Design review of the part shown in the three views and the two pictorial views. Dimensions are in mm from the part's minimum x, y and z. A direction names the side the tool comes from. Give positions to 0.01 mm unless a question says otherwise; leave off trailing zeros. Loops run counter-clockwise (first coordinate to the right, second up) from the corner with the lowest first, then second, coordinate; pieces in that order, holes last. Notation, with made-up numbers: (-26.75, 32) -> (31.25, 32) arc R21 ccw to (31.25, 65) -> close; hole circle Ø6 at (83.5, 1). An arc over 180 degrees is marked (long way). One line per question, with ' | ' between items. Start each with the question number.
(1) Consider section B-B (y = 3). Write out the cut boundary in (x, z).
(2) Insertion check: P1, Ø1.5, axis at x = 10, y = 2, coming from the -Z side; P2, Ø2, axis at x = 3.5, z = 2.5, coming from the -Y side. Each pin has a flat end and moves straight along its axis. Give the tip position at first contact, or say it passes through.
(3) Tool access review of the marked faces 1 and 2: name each direction out of +Z, -Z, +X, -X, +Y, -Y from which nothing blocks a thin tool from reaching the whole face with its end or side.
(4) Consider section C-C (y = 6). Write out the cut boundary in (x, z).
(5) Wall thickness on probe 1 along Y at (x, z) = (7.75, 10.25); probe 2 along Z at (x, y) = (5.5, 4.75); probe 3 along Y at (x, z) = (1.25, 8.75): over which ranges is each line inside the solid? List them lowest first.
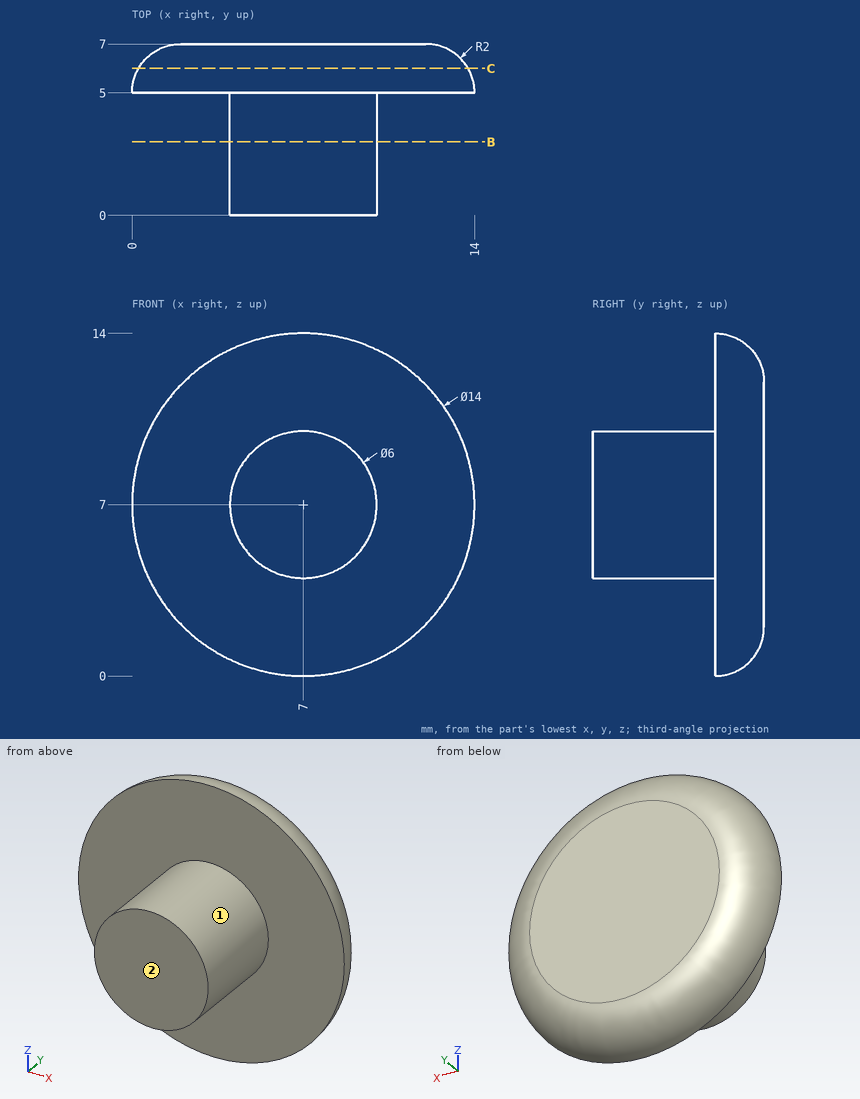
A:
1) outline: circle Ø6 at (7, 7)
2) P1: stops at z = 5.02 | P2: stops at y = 5
3) face 1: -Y | face 2: +Z, -Z, +X, -X, -Y
4) outline: circle Ø13.46 at (7, 7)
5) probe 1: y = 5 to 7 | probe 2: z = 4.4 to 9.6 | probe 3: y = 5 to 6.73
